Geometry: final body of the model. Coordinates: model frame, mm. A direction names the side the tool comes from. Give positions to 0.01 mm unless a question says otherwise; leave off trailing zeros. Loops run counter-clockwise (first coordinate to the right, second up) from the corner with the lowest first, then second, coordinate; pieces in that order, holes last.
```python
from build123d import *

# Parameters (mm, degrees)
SKETCH1_W           = 47
SKETCH1_H           = 69
BOSS_EXTRUDE1_DEPTH = 2
FILLET1_R           = 7
SKETCH2_W           = 20
SKETCH2_H           = 14
SKETCH2_H_2         = 21.8
CUT_EXTRUDE1_DEPTH  = 2
FILLET2_R           = 4
SKETCH4_W           = 3.5
SKETCH4_H           = 19.5
BOSS_EXTRUDE2_DEPTH = 6
FILLET3_START       = -210.696929932
FILLET3_DEPTH       = 43.606418674
FILLET3_2_DEPTH     = 3.5
FILLET3_START_2     = -170.590511258
FILLET3_3_DEPTH     = 3.5
SKETCH5_R           = 1
CUT_EXTRUDE2_DEPTH  = 445.178336025


with BuildPart() as part:
    # Sketch1 → Boss-Extrude1 (new body)
    with BuildSketch(Plane.XY.offset(10)):
        with Locations((-188.893720595, 406.995202033)):
            Rectangle(SKETCH1_W, SKETCH1_H)
    extrude(amount=BOSS_EXTRUDE1_DEPTH)

    # Fillet1
    fillet1_edges = [part.edges().sort_by_distance(p)[0] for p in [
        (-212.393720595, 441.495202033, 11),
        (-165.393720595, 441.495202033, 11),
        (-165.393720595, 372.495202033, 11),
        (-212.393720595, 372.495202033, 11),
    ]]
    fillet(fillet1_edges, radius=FILLET1_R)

    # Sketch2 → Cut-Extrude1 (cut)
    with BuildSketch(Plane.XY.offset(12)):
        with Locations((-190.900590621, 424.93058769)):
            Rectangle(SKETCH2_W, SKETCH2_H)
        with Locations((-190.900590621, 393.92847215)):
            Rectangle(SKETCH2_W, SKETCH2_H_2)
    extrude(amount=-CUT_EXTRUDE1_DEPTH, mode=Mode.SUBTRACT)

    # Fillet2
    fillet2_edges = [part.edges().sort_by_distance(p)[0] for p in [
        (-200.900590621, 417.93058769, 11),
        (-200.900590621, 431.93058769, 11),
        (-180.900590621, 431.93058769, 11),
        (-180.900590621, 417.93058769, 11),
        (-200.900590621, 383.02847215, 11),
        (-200.900590621, 404.82847215, 11),
        (-180.900590621, 404.82847215, 11),
        (-180.900590621, 383.02847215, 11),
    ]]
    fillet(fillet2_edges, radius=FILLET2_R)

    # Sketch4 → Boss-Extrude2 (add)
    with BuildSketch(Plane.XY.offset(12)):
        with Locations((-168.840511258, 411.411865234)):
            Rectangle(SKETCH4_W, SKETCH4_H)
        with Locations((-208.946929932, 411.411865234)):
            Rectangle(SKETCH4_W, SKETCH4_H)
    extrude(amount=BOSS_EXTRUDE2_DEPTH)

    # Fillet3: read off the stored shape, not the designer's step
    # Fillet3 outline → Fillet3 (cut)
    with BuildSketch(Plane.YZ.offset(FILLET3_START)):
        with BuildLine():
            ThreePointArc((418.161865234, 18), (420.283185578, 17.121320344), (421.161865234, 15))
            Line((421.161865234, 15), (421.161865234, 18))
            Line((421.161865234, 18), (418.161865234, 18))
        make_face()
        with BuildLine():
            ThreePointArc((401.661865234, 15), (402.540544891, 17.121320343), (404.661865234, 18))
            Line((404.661865234, 18), (401.661865234, 18))
            Line((401.661865234, 18), (401.661865234, 15))
        make_face()
    extrude(amount=FILLET3_DEPTH, mode=Mode.SUBTRACT)

    # Fillet3 2 outline → Fillet3 2 (add)
    with BuildSketch(Plane.YZ.offset(FILLET3_START)):
        with BuildLine():
            Line((421.161865234, 12), (424.161865234, 12))
            ThreePointArc((424.161865234, 12), (422.040544891, 12.878679657), (421.161865234, 15))
            Line((421.161865234, 15), (421.161865234, 12))
        make_face()
        with BuildLine():
            Line((398.661865234, 12), (401.661865234, 12))
            Line((401.661865234, 12), (401.661865234, 15))
            ThreePointArc((401.661865234, 15), (400.783185578, 12.878679656), (398.661865234, 12))
        make_face()
    extrude(amount=FILLET3_2_DEPTH)

    # Fillet3 3 outline → Fillet3 3 (add)
    with BuildSketch(Plane.YZ.offset(FILLET3_START_2)):
        with BuildLine():
            Line((421.161865234, 12), (424.161865234, 12))
            ThreePointArc((424.161865234, 12), (422.040544891, 12.878679657), (421.161865234, 15))
            Line((421.161865234, 15), (421.161865234, 12))
        make_face()
        with BuildLine():
            Line((398.661865234, 12), (401.661865234, 12))
            Line((401.661865234, 12), (401.661865234, 15))
            ThreePointArc((401.661865234, 15), (400.783185578, 12.878679656), (398.661865234, 12))
        make_face()
    extrude(amount=FILLET3_3_DEPTH)

    # Sketch5 → Cut-Extrude2 (cut, through all)
    with BuildSketch(Plane(origin=(-167.090511258, 0, 0), x_dir=(0, 0, -1), z_dir=(1, 0, 0))):
        with Locations((-15.033399781, 407.479533559)):
            Circle(SKETCH5_R)
        with Locations((-15.033399781, 415.979533559)):
            Circle(SKETCH5_R)
    extrude(amount=-CUT_EXTRUDE2_DEPTH, mode=Mode.SUBTRACT)


solid = part.part
```
Q1. Material intervals for probe 1 along X at (y, z) = (420.5, 14.25); probe 2 along Z at (x, y) = (-174.5, 382); probe 3 along X at (y, z) = (430.5, 11.5), sorted ascending.
Q2. Reachability of faces 1 (the face through (-189, 372.495, 11)), 2 (the face through (-209, 412, 18)), 3 (the face through (-167.091, 411, 15)), 4 (the face through (-180.901, 425, 11)), 5 (the face through (-207.197, 411, 15)) from +Z, -Z, +X, -X, +Y, -Y: full face, straight path, thin tool, end or side. Return the list, or none.
Q3. Section query B-B, the plane x = -188. Return loops of the section in (y, z).
Q4. Mould query, pull axis Z, two halves, no side actions, for faces 6 (the face through (-189, 407, 12)), 7 (the face through (-208.92, 408.47, 15.16)), 8 (the face through (-199.7, 430.79, 10.99)). Classes: +Z half, -Z half, draft (parallel to the pull), parting line (faces both ways), or undercut.
Q5. Section query D-D, the plane y = 411.5. Return loops of the section in (x, z), and give its area (3 significant figures).
Q6. Section query A-A, the plane y = 426. Return loops of the section in (x, z).
Q7. Pin query (flat end, axial travel): pin 1 Ø1.6 at (y, z) = (415.98, 15.03) entering from -X; pin 2 Ø3 at (y, z) = (416, 14) entering from +X; pin 3 Ø3 at (y, z) = (412.5, 15.5) entering from -X. Return the tip coordinate at first contact, or that it passes through.
Q8. Section query C-C, the plane z = 17. Return loops of the section in (x, y).
Resolved:
1. probe 1: x = -210.7 to -207.2, -170.59 to -167.09
1. probe 2: z = 10 to 12
1. probe 3: x = -212.39 to -199.97, -181.83 to -165.39
2. face 1: +Z, -Z, +X, -X, -Y
2. face 2: +Z, +X, -X, +Y, -Y
2. face 3: +Z, +X, +Y, -Y
2. face 4: +Z, -Z
2. face 5: +Z, +Y, -Y
3. outline: (372.5, 10) - (383.03, 10) - (383.03, 12) - (372.5, 12) - close; (404.83, 10) - (417.93, 10) - (417.93, 12) - (404.83, 12) - close; (431.93, 10) - (441.5, 10) - (441.5, 12) - (431.93, 12) - close
4. face 6: +Z half
4. face 7: undercut
4. face 8: draft
5. outline: (-212.39, 10) - (-165.39, 10) - (-165.39, 12) - (-167.09, 12) - (-167.09, 18) - (-170.59, 18) - (-170.59, 12) - (-207.2, 12) - (-207.2, 18) - (-210.7, 18) - (-210.7, 12) - (-212.39, 12) - close
5. area: 136 mm2
6. outline: (-212.39, 10) - (-200.9, 10) - (-200.9, 12) - (-212.39, 12) - close; (-180.9, 10) - (-165.39, 10) - (-165.39, 12) - (-180.9, 12) - close
7. pin 1: passes through
7. pin 2: stops at x = -167.09
7. pin 3: stops at x = -210.7
8. outline: (-210.7, 402.43) - (-207.2, 402.43) - (-207.2, 420.4) - (-210.7, 420.4) - close; (-170.59, 402.43) - (-167.09, 402.43) - (-167.09, 420.4) - (-170.59, 420.4) - close
